from build123d import *

# Parameters (mm, degrees)
F0_W     = 47.5
F0_H     = 2
F0_W_2   = 2
F0_W_3   = 2.25
F0_H_2   = 13.5
F0_W_4   = 56
F0_H_3   = 9.5
F1_DEPTH = 25
F2_W     = 6.25
F2_H     = 2
F3_DEPTH = 25
F4_W     = 51.5
F4_H     = 9.5
F5_DEPTH = 2


with BuildPart() as f1:
    # F0 (on Front) → F1 (new body)
    with BuildSketch(Plane.XZ):
        with Locations((23.75, 10.5)):
            Rectangle(F0_W, F0_H)
        with Locations((-1, 10.5)):
            Rectangle(F0_W_2, F0_H)
        Polygon((-2, 0), (0, 0), (0, 9.5), (-2, 9.5), (-2, 2), align=None)
        with Locations((-3.125, 1)):
            Rectangle(F0_W_3, F0_H)
        with Locations((-5.25, 1)):
            Rectangle(F0_W_2, F0_H)
        with Locations((-5.25, -6.75)):
            Rectangle(F0_W_2, F0_H_2)
        with Locations((-5.25, -14.5)):
            Rectangle(F0_W_2, F0_H)
        with Locations((23.75, -14.5)):
            Rectangle(F0_W_4, F0_H)
        with Locations((52.75, -14.5)):
            Rectangle(F0_W_2, F0_H)
        with Locations((52.75, -6.75)):
            Rectangle(F0_W_2, F0_H_2)
        with Locations((52.75, 1)):
            Rectangle(F0_W_2, F0_H)
        with Locations((48.5, 4.75)):
            Rectangle(F0_W_2, F0_H_3)
        with Locations((48.5, 10.5)):
            Rectangle(F0_W_2, F0_H)
    extrude(amount=F1_DEPTH)

    # F2 (on face) → F3 (join)
    with BuildSketch(Plane.XZ.offset(25)):
        with Locations((50.625, 1)):
            Rectangle(F2_W, F2_H)
    extrude(amount=-F3_DEPTH)

    # F4 (on face) → F5 (join)
    with BuildSketch(Plane.XZ.offset(25)):
        Polygon((-6.25, 2), (-6.25, -15.5), (53.75, -15.5), (53.75, 2), (49.5, 2), (-2, 2), align=None)
        with Locations((23.75, 6.75)):
            Rectangle(F4_W, F4_H)
    extrude(amount=F5_DEPTH)


solid = f1.part
Model file for the job. Use its own axes, mm. A direction names the side the tool comes from. Give positions to 0.01 mm unless a question says otherwise; leave off trailing zeros. Write each loop counter-clockwise with the first axis right and the second up, starting at its lowest first coordinate (ties: lowest second). Pieces come first, ordered by that corner, then holes. Notation, with made-up numbers: M 12,12 L 56,12 A16 cw 56,38 Z; hole C 12.25,17.25 d11. An arc over 180 degrees is marked long. One line per item, written item: value. Start each with the question number.
Q1. Probe probe 1 along X at (y, z) = (-4.75, 2.5); probe 2 along Z at (x, y) = (2.5, -24.25); probe 3 along X at (y, z) = (-7, -4.25). List the from-to ranges inside material, lowest first. Write a range as [from, to].
Q2. Saw through at C-C, the plane x = 13. Write the cut outline in (y, z).
Q3. Saw through at B-B, the plane y = -24.25. Write the cut outline in (x, z).
Q4. 3-axis set-ups, long thin cutter, end or side, ignore diameter. For faces 4 (the flat face through (-2, -13, 7)), 5 (the flat face through (-6.25, -13, -7)), 6 (the flat face through (52, -13, 2)), 7 (the flat face through (51.75, -12, -7)): which of +Z, -Z, +X, -X, +Y, -Y reach the whole face in a straight line?
Q5. Drop flat-ended pins along their axis: pin 1 Ø3 at (y, z) = (-9, 9) entering from -X; pin 2 Ø1 at (x, z) = (37, 0.5) entering from +Y; pin 3 Ø1.3 at (x, y) = (-5, -20) entering from +Z. Give the stop position or say it passes through.
Q6. Two-plate mould, pull along Z, no slides. Class faces 1 (the flat face through (23, -13, -15.5)), 2 (the flat face through (53.75, -13, -7)), 3 (the flat face through (24, -12, -13.5)): +Z half, -Z half, draft (parallel to the pull), parting line (faces both ways), or undercut.
Q7. Saw through at A-A, the plane z = 4. Write the cut outline in (x, y), plus the area to 3 significant figures.
Output values:
1. probe 1: x = [-2, 0], [47.5, 49.5]
1. probe 2: z = [-15.5, -13.5], [9.5, 11.5]
1. probe 3: x = [-6.25, -4.25], [51.75, 53.75]
2. outline: M -27,-15.5 L 0,-15.5 L 0,-13.5 L -25,-13.5 L -25,9.5 L 0,9.5 L 0,11.5 L -27,11.5 Z
3. outline: M -6.25,-15.5 L 53.75,-15.5 L 53.75,2 L 49.5,2 L 49.5,11.5 L -2,11.5 L -2,2 L -6.25,2 Z; hole M -4.25,-13.5 L 51.75,-13.5 L 51.75,0 L 47.5,0 L 47.5,9.5 L 0,9.5 L 0,0 L -4.25,0 Z
4. face 4: +Z, -X, +Y, -Y
4. face 5: +Z, -Z, -X, +Y, -Y
4. face 6: +Z, +X, +Y, -Y
4. face 7: +Y
5. pin 1: stops at x = -2
5. pin 2: stops at y = -25
5. pin 3: stops at z = 2
6. face 1: -Z half
6. face 2: draft
6. face 3: undercut
7. outline: M -2,-27 L 49.5,-27 L 49.5,0 L 47.5,0 L 47.5,-25 L 0,-25 L 0,0 L -2,0 Z
7. area: 203 mm²
